Can you work these out from the model? Positions are in its coordinate system, mm. A direction names the side the tool comes from. Give positions to 0.01 mm unless a question says otherwise; leave off trailing zeros. Order: outer loops, then holes, each group sorted by start corner. A loop starts at its lowest first (then second) coordinate and runs counter-clockwise, first axis right, second up. Notation, with made-up numbers: (26, 82.5) - (44, 82.5) arc R29 cw to (44, 102.5) - close; hole circle Ø4 at (29, 27). An arc over 180 degrees is marked (long way). Use one line per item in the form item = value. Start each with the question number.
1) Which directions (+Z, -Z, +X, -X, +Y, -Y) give clear straight access to the entire face, cutting with the end or side of a thin tool? Please do faces 1 (the flat face through (-26.9, 4.4, 13.3)), 2 (the flat face through (-25.5, -15, -5)), 3 (the flat face through (-13.8, -6, 15)).
2) Please list where these lines run through material, in increasing order: probe 1 along Z at (x, y) = (-17.5, 0); probe 2 along X at (y, z) = (-10.5, -11); probe 3 along Z at (x, y) = (-6.75, 0).
3) Suppose I cut it at C-C, the plane x = -19.5. Write out the boundary of the cut face in (y, z).
4) Suppose I cut it at D-D, the plane x = -9. Write out the boundary of the cut face in (y, z), and give its area (3 significant figures).
5) Suppose I cut it at A-A, the plane y = 0. Write out the boundary of the cut face in (x, z).
6) We'd pull the mould along Z, two halves only. Please class faces 4 (the conical face through (-6.997, 15.184, -3.372)), 5 (the flat face through (0, -14, 2)), 6 (the cylindrical face through (-13.26, 13.21, 4.16)): released by +Z, released by -Z, zero draft, split by the parting line, or undercut.
7) For pin 1 (10 mm diameter, centred on x = -23.5, z = -9.5, fed in from +Y); pin 2 (1.5 mm diameter, centred on y = 11, z = -7, fed in from -X); pin 3 (1 mm diameter, centred on x = -5.5, z = -3.5, fed in from +Y); pin 4 (1.5 mm diameter, centred on x = -16.5, y = 10, fed in from +Z), each with a flat end and sliding along its axis, tell me the tip position at first contact or that it passes through.
```python
from build123d import *

# Parameters (mm, degrees)
F2_R     = 13.85
F3_DEPTH = 26.901
F4_R     = 16.4
F4_R_2   = 15.05
F5_DEPTH = 1.4


with BuildPart() as f1:
    # F0 (on Front) → F1 (revolve)
    with BuildSketch(Plane.XZ):
        Polygon((-13.8, 16.4), (-26.9, 16.4), (-26.9, 0), (-13.8, 0), (-13.8, 15.8), align=None)
        Polygon((0, 15.3), (-13.8, 15.8), (-13.8, 0), (0, 0), align=None)
    revolve(axis=Axis((-20.35, 0, 0), (1, 0, 0)))

    # F2 (on face) → F3 (cut, through all)
    with BuildSketch(Plane.YZ):
        Circle(F2_R)
    extrude(amount=-F3_DEPTH, mode=Mode.SUBTRACT)

    # F4 (on face) → F5 (cut)
    with BuildSketch(Plane(origin=(-26.9, 0, 0), x_dir=(0, -1, 0), z_dir=(-1, 0, 0))):
        Circle(F4_R)
        Circle(F4_R_2, mode=Mode.SUBTRACT)
    extrude(amount=-F5_DEPTH, mode=Mode.SUBTRACT)


solid = f1.part
```
Result sheet:
q1.face_1 = +Z, -Z, -X, +Y, -Y
q1.face_2 = -X
q1.face_3 = +X
q2.probe_1 = -16.4 to -13.85, 13.85 to 16.4
q2.probe_2 = -25.5 to 0
q2.probe_3 = -15.54 to -13.85, 13.85 to 15.54
q3.outline = circle Ø32.8 at (0, 0); hole circle Ø27.7 at (0, 0)
q4.outline = circle Ø31.25 at (0, 0); hole circle Ø27.7 at (0, 0)
q4.area = 164 mm²
q5.outline = (-26.9, -15.05) - (-25.5, -15.05) - (-25.5, -16.4) - (-13.8, -16.4) - (-13.8, -15.8) - (0, -15.3) - (0, -13.85) - (-26.9, -13.85) - close; (-26.9, 13.85) - (0, 13.85) - (0, 15.3) - (-13.8, 15.8) - (-13.8, 16.4) - (-25.5, 16.4) - (-25.5, 15.05) - (-26.9, 15.05) - close
q6.face_4 = split by the parting line
q6.face_5 = zero draft
q6.face_6 = undercut
q7.pin_1 = 15.77
q7.pin_2 = through
q7.pin_3 = 15.21
q7.pin_4 = 13.54
